from build123d import *

# Parameters (mm, degrees)
CROQUIS1_R              = 1.5
CROQUIS1_R_2            = 3
CROQUIS1_R_3            = 3.4
SALIENTE_EXTRUIR1_DEPTH = 6


with BuildPart() as part:
    # Croquis1 → Saliente-Extruir1 (new body)
    with BuildSketch(Plane.XY):
        with BuildLine():
            Line((8.1e-08, 14.249999874), (8.1e-08, 2.999999874))
            ThreePointArc((8.1e-08, 2.999999874), (0.878679737, 0.87867953), (3.000000081, -1.26e-07))
            Line((3.000000081, -1.26e-07), (18.000000081, -1.26e-07))
            Line((18.000000081, -1.26e-07), (40.911193324, 34.196329551))
            ThreePointArc((40.911193324, 34.196329551), (41.527076457, 35.020483475), (42.224381081, 35.776993874))
            Line((42.224381081, 35.776993874), (98.096843081, 90.459473874))
            ThreePointArc((98.096843081, 90.459473874), (108.550843923, 98.63680641), (120.546851363, 104.315776961))
            ThreePointArc((120.546851363, 104.315776961), (125.500442362, 107.172433842), (129.025046114, 111.675290792))
            Line((129.025046114, 111.675290792), (138.514418989, 130.248169023))
            ThreePointArc((138.514418989, 130.248169023), (137.107819922, 139.483655494), (127.90475, 141.088721))
            Line((127.90475, 141.088721), (109.131917, 132.001327))
            ThreePointArc((109.131917, 132.001327), (104.554236665, 128.574463552), (101.591616002, 123.683509744))
            ThreePointArc((101.591616002, 123.683509744), (95.655747756, 111.812521161), (87.255287964, 101.536959032))
            Line((87.255287964, 101.536959032), (30.072463964, 45.572027032))
            ThreePointArc((30.072463964, 45.572027032), (29.779023988, 45.268761189), (29.502525894, 44.949972866))
            Line((29.502525894, 44.949972866), (15.949120522, 28.43588954))
            ThreePointArc((15.949120522, 28.43588954), (12.726828906, 25.305121034), (8.887000234, 22.972613701))
            ThreePointArc((8.887000234, 22.972613701), (6.271558617, 21.381766549), (4.079708958, 19.244683353))
            Line((4.079708958, 19.244683353), (8.1e-08, 14.249999874))
        make_face()
        with Locations((25.371621, 27.641642)):
            Circle(CROQUIS1_R, mode=Mode.SUBTRACT)
        with Locations((35.493241781, 40.03328422)):
            Circle(CROQUIS1_R, mode=Mode.SUBTRACT)
        with Locations((15.25, 15.25)):
            Circle(CROQUIS1_R_2, mode=Mode.SUBTRACT)
        with Locations((115.667525989, 118.500000023)):
            Circle(CROQUIS1_R_3, mode=Mode.SUBTRACT)
        with BuildLine():
            Line((105.901407198, 117.055029782), (107.901292, 117.033504))
            ThreePointArc((107.901292, 117.033504), (109.4678845, 118.5667315), (107.934657, 120.133324))
            Line((107.934657, 120.133324), (105.934773, 120.15485))
            ThreePointArc((105.934773, 120.15485), (104.368758386, 118.621616566), (105.901407198, 117.055029782))
        make_face(mode=Mode.SUBTRACT)
        with BuildLine():
            Line((114.012675, 108.767248), (114.034201, 110.767132))
            ThreePointArc((114.034201, 110.767132), (115.6007945, 112.3003595), (117.134022, 110.733766))
            Line((117.134022, 110.733766), (117.112495218, 108.733882198))
            ThreePointArc((117.112495218, 108.733882198), (115.545908434, 107.201233386), (114.012675, 108.767248))
        make_face(mode=Mode.SUBTRACT)
        with BuildLine():
            Line((124.211353692, 123.893635573), (128.262273986, 123.850032801))
            ThreePointArc((128.262273986, 123.850032801), (130.375033742, 124.426891571), (131.867331288, 126.029878739))
            Line((131.867331288, 126.029878739), (134.952413288, 132.068090739))
            ThreePointArc((134.952413288, 132.068090739), (134.24911451, 136.685834372), (129.647579323, 137.48836746))
            Line((129.647579323, 137.48836746), (123.544360208, 134.533971661))
            ThreePointArc((123.544360208, 134.533971661), (121.909622476, 133.076524245), (121.287419986, 130.976670801))
            Line((121.287419986, 130.976670801), (121.243816986, 126.925750801))
            ThreePointArc((121.243816986, 126.925750801), (122.099613791, 124.795096288), (124.211353692, 123.893635573))
        make_face(mode=Mode.SUBTRACT)
        with BuildLine():
            Line((125.400278, 116.84515), (123.400394, 116.866676))
            ThreePointArc((123.400394, 116.866676), (121.867759233, 118.43326212), (123.433759, 119.966496))
            Line((123.433759, 119.966496), (125.433643802, 119.944970218))
            ThreePointArc((125.433643802, 119.944970218), (126.96687101, 118.378377208), (125.400278, 116.84515))
        make_face(mode=Mode.SUBTRACT)
        with BuildLine():
            Line((117.322376, 128.232752), (117.30085, 126.232868))
            ThreePointArc((117.30085, 126.232868), (115.734268362, 124.700742507), (114.201029, 126.266234))
            Line((114.201029, 126.266234), (114.222555782, 128.266117802))
            ThreePointArc((114.222555782, 128.266117802), (115.789148792, 129.79934501), (117.322376, 128.232752))
        make_face(mode=Mode.SUBTRACT)
    extrude(amount=SALIENTE_EXTRUIR1_DEPTH)


solid = part.part
The listing builds one solid part. Answer for the finished solid, in the listing's coordinates (mm). A direction names the side the tool comes from. Round coordinates to 2 decimals unless told otherwise and drop trailing zeros. Order: outer loops, then holes, each group sorted by start corner. A loop starts at its lowest first (then second) coordinate and runs counter-clockwise, first axis right, second up. Notation, with made-up numbers: M 22,17 L 68,17 A22 cw 68,41 Z; hole C 70.25,65.5 d2. An arc over 180 degrees is marked long. Answer in a Markdown table with one row per item. Add a question column.
1) Which of the six approach directions +Z, -Z, +X, -X, +Y, -Y give full straight-line access (tool end or side, diameter ignored) to faces 4 (the face through (133.703, 120.832, 2.958)), 5 (the face through (126.639, 136.032, 2.958))?
2) The part is cut by section C-C on x = 74.5. Determine the outline of the cut face in (y, z), plus the area to 3 significant figures.
3) The part is cut by section A-A on z = 3.25. Count the separate pieces of the cut face and the enclosed holes in it, plus the area to 3 significant figures.
4) Consider line 1 along Y through (x, z) = (116, 2.6); line 2 along Y through (x, z) = (15.25, 2); line 3 along X through (y, z) = (121.5, 4.3). Determine where each line is inside the solid, lowest interval first. Write a range as from..to.
5) Determine the mould class of faces 1 (the face through (22.82, 36.81, 2.96)), 2 (the face through (69, 71, 0)), 3 (the face through (104.37, 118.66, 2.96)) for opening direction Y: pulls with the +Y half, pulls with the -Y half, needs draft (parallel to the pull), parting line crosses it, or undercut.
6) Flat-ended cylindrical pins translate along their axes: pin 1 Ø2.5 at (x, y) = (35.49, 40.03) entering from -Z (3 decimals); pin 2 Ø2 at (x, z) = (92.5, 0.5) entering from +Y; pin 3 Ø9.5 at (x, y) = (15.25, 15.25) entering from +Z; pin 4 Ø1.5 at (y, z) = (109.5, 4.5) entering from -X. Find the tip coordinate at first contact, or state that the pin passes through.
7) The part is cut by section B-B on y = 63.5. Determine the outline of the cut face in (x, z), plus the area to 3 significant figures.
Findings below:
| question | item | result |
|---|---|---|
| 1 | face 4 | +Z, -Z, +X, -Y |
| 1 | face 5 | +Z, -Z |
| 2 | outline | M 67.37,0 L 89.05,0 L 89.05,6 L 67.37,6 Z |
| 2 | area | 130 mm² |
| 3 | separate pieces | 1 |
| 3 | enclosed holes | 9 |
| 3 | area | 3,190 mm² |
| 4 | line 1 | y = 102.54..107.26, 112.24..115.12, 121.88..124.72, 129.78..135.33 |
| 4 | line 2 | y = 0..12.25, 18.25..27.63 |
| 4 | line 3 | x = 100.74..114.07, 117.27..134.04 |
| 5 | face 1 | pulls with the +Y half |
| 5 | face 2 | needs draft |
| 5 | face 3 | undercut |
| 6 | pin 1 | passes through |
| 6 | pin 2 | stops at y = 108.7 |
| 6 | pin 3 | stops at z = 6 |
| 6 | pin 4 | stops at x = 93.54 |
| 7 | outline | M 48.39,0 L 70.55,0 L 70.55,6 L 48.39,6 Z |
| 7 | area | 133 mm² |
